```python
from build123d import *

# Parameters (mm, degrees)
ESTRUSIONE_ESTRUSIONE1_DEPTH = 4
RACCORDO1_R                  = 10
RACCORDO2_R                  = 4
RACCORDO9_R                  = 3
RACCORDO10_R                 = 3
RACCORDO11_R                 = 5


with BuildPart() as part:
    # Schizzo1 → Estrusione-Estrusione1 (new body)
    with BuildSketch(Plane(origin=(0, 0, 0), x_dir=(1, 0, 0), z_dir=(0, 1, 0))):
        Polygon((-11.4, 23), (-11.4, 13), (-5.4, 13), (-5.4, 16), (0, 16), (0, 0), (110, 0), (110, 16), (115.4, 16), (115.4, 13), (121.4, 13), (121.4, 23), (110, 23), (110, 26), (95, 26), (95, 17), (15, 17), (15, 26), (0, 26), (0, 23), align=None)
    extrude(amount=ESTRUSIONE_ESTRUSIONE1_DEPTH)

    # Raccordo1
    # the kernel refuses this fillet: 10 mm, written as the material it takes off along each edge
    with BuildSketch(Plane(origin=(95, -24.874685928, -26), x_dir=(1, 0, 0), z_dir=(0, 1, 0))) as raccordo1_piece_1:
        with BuildLine():
            CenterArc((9.949874371, -10), RACCORDO1_R, 90, 84.260829523)
            Line((0, -9), (-0.198997487, -8.98))
            ThreePointArc((-0.198997487, -8.98), (-0.2, -4.5), (-0.2, 0))
            Line((-0.2, 0), (0, 0.2))
            Line((0, 0.2), (9.949874371, 0.2))
            Line((9.949874371, 0.2), (9.949874371, 0))
        make_face()
    extrude(amount=53.749371855, mode=Mode.SUBTRACT)
    with BuildSketch(Plane(origin=(15, -24.874685928, -26), x_dir=(0, 0, 1), z_dir=(0, 1, 0))) as raccordo1_piece_2:
        with BuildLine():
            CenterArc((10, -9.949874371), RACCORDO1_R, 95.739170477, 84.260829523)
            Line((0, -9.949874371), (-0.2, -9.949874371))
            Line((-0.2, -9.949874371), (-0.2, 0))
            Line((-0.2, 0), (0, 0.2))
            ThreePointArc((0, 0.2), (4.5, 0.2), (8.98, 0.198997487))
            Line((8.98, 0.198997487), (9, 0))
        make_face()
    extrude(amount=53.749371855, mode=Mode.SUBTRACT)

    # Raccordo2
    raccordo2_edges = [part.edges().sort_by_distance(p)[0] for p in [
        (110, 2, 0),
        (0, 2, 0),
    ]]
    fillet(raccordo2_edges, radius=RACCORDO2_R)

    # Raccordo9
    raccordo9_edges = [part.edges().sort_by_distance(p)[0] for p in [
        (-11.4, 2, -13),
        (-11.4, 2, -23),
    ]]
    fillet(raccordo9_edges, radius=RACCORDO9_R)

    # Raccordo10
    raccordo10_edges = [part.edges().sort_by_distance(p)[0] for p in [
        (121.4, 2, -23),
        (121.4, 2, -13),
    ]]
    fillet(raccordo10_edges, radius=RACCORDO10_R)

    # Raccordo11
    raccordo11_edges = [part.edges().sort_by_distance(p)[0] for p in [
        (15, 2, -17),
        (95, 2, -17),
    ]]
    fillet(raccordo11_edges, radius=RACCORDO11_R)


solid = part.part
```
Work out the finished part from the listing and answer in its coordinate system (mm). A direction names the side the tool comes from. Give positions to 0.01 mm unless a question says otherwise; leave off trailing zeros. Loops run counter-clockwise (first coordinate to the right, second up) from the corner with the lowest first, then second, coordinate; pieces in that order, holes last. Notation, with made-up numbers: (79, -21.5) -> (85, -21.5) arc R19 cw to (85, -0.5) -> close; hole circle Ø2 at (-20, -24.75). An arc over 180 degrees is marked (long way). Write item = value, one per line. Start each with the question number.
(1) Find section D-D on z = -6.25. Give the vertices of the cut face in (x, y).
(2) Given pin 1 Ø0.9 at (y, z) = (1.5, -24.5) entering from +X; pin 2 Ø2 at (x, y) = (116, 3) entering from -Z; pin 3 Ø2 at (x, y) = (40.5, 2.5) entering from -Z, each flat-ended and moving along its own axis, determine where each tip first touches the part or whether it passes through.
(3) The mould has two halves that part along X. Classify faces 5 (the flat face through (54, 2, 0)), 6 (the flat face through (-5.4, 2, -14)), 7 (the cylindrical face through (120.54, 2.03, -22.1)): +X half, -X half, draft (parallel to the pull), parting line (faces both ways), or undercut.
(4) Find section A-A on y = 1.25. Give the vertices of the cut face in (x, z), and give its area (3 significant figures).
(5) Find section B-B on z = -18.5. Give the vertices of the cut face in (x, y).
(6) Find section C-C on x = 70. Give the vertices of the cut face in (y, z).
(7) Which of the six approach directions +Z, -Z, +X, -X, +Y, -Y give full straight-line access (tool end or side, diameter ignored) to faces 1 (the flat face through (115.4, 2, -15)), 2 (the flat face through (117, 2, -13)), 3 (the flat face through (-7, 2, -13)), 4 (the cylindrical face through (99.54, 1.97, -24.41))?
(8) Find the intervals of material crossed by probe 1 along X at (y, z) = (3, -14.75); probe 2 along X at (y, z) = (2.6, -11.5); probe 3 along Z at (x, y) = (84, 2.7), in increasing order. Write a range as from..to.
From the geometry:
q1.outline = (0, 0) -> (110, 0) -> (110, 4) -> (0, 4) -> close
q2.pin_1 = 110
q2.pin_2 = -23
q2.pin_3 = -17
q3.face_5 = draft
q3.face_6 = undercut
q3.face_7 = +X half
q4.outline = (-11.4, -20) arc R3 ccw to (-8.4, -23) -> (0, -23) -> (0, -26) -> (5.05, -26) arc R10 ccw to (14.22, -20) arc R5 cw to (18.8, -17) -> (91.2, -17) arc R5 cw to (95.78, -20) arc R10 ccw to (104.95, -26) -> (110, -26) -> (110, -23) -> (118.4, -23) arc R3 ccw to (121.4, -20) -> (121.4, -16) arc R3 ccw to (118.4, -13) -> (115.4, -13) -> (115.4, -16) -> (110, -16) -> (110, -4) arc R4 ccw to (106, 0) -> (4, 0) arc R4 ccw to (0, -4) -> (0, -16) -> (-5.4, -16) -> (-5.4, -13) -> (-8.4, -13) arc R3 ccw to (-11.4, -16) -> close
q4.area = 2,280 mm^2
q5.outline = (-11.4, 0) -> (15.23, 0) -> (15.23, 4) -> (-11.4, 4) -> close; (94.77, 0) -> (121.4, 0) -> (121.4, 4) -> (94.77, 4) -> close
q6.outline = (0, -17) -> (4, -17) -> (4, 0) -> (0, 0) -> close
q7.face_1 = +Z, +Y, -Y
q7.face_2 = +Z, +X, +Y, -Y
q7.face_3 = +Z, -X, +Y, -Y
q7.face_4 = -Z, +Y, -Y
q8.probe_1 = -11.13..-5.4, 0..110, 115.4..121.13
q8.probe_2 = 0..110
q8.probe_3 = -17..0
